Check sheet for the modelled part. Datum: model origin and axes. Units: mm. Round coordinates to 2 decimals unless told otherwise and drop trailing zeros. Loops run counter-clockwise (first coordinate to the right, second up) from the corner with the lowest first, then second, coordinate; pieces in that order, holes last. Notation, with made-up numbers: (41.5, 0) - (49.5, 0) arc R17 cw to (49.5, 29) - close; hole circle Ø11 at (-9.5, 38.25). An arc over 180 degrees is marked (long way). Put each result on its own line as item: value. Start each with the question number.
Item 1: Material ranges on line 1 along X through (y, z) = (2.9, 110); line 2 along X through (y, z) = (11.75, 110); line 3 along Z through (x, y) = (235, 3.95), recorded low to high.
Item 2: Section check B-B, the plane x = 169.5. Record the cut outline in (y, z), and give its area (3 significant figures).
Item 3: Section check C-C, the plane z = 136. Record the cut outline in (x, y).
Item 4: Section check A-A, the plane y = 12.75. Give the number of separate pieces and of enclosed holes in the cut face, and give its area (3 significant figures).
Item 5: Gauge pin test, flat ends, axial feed: pin 1 Ø8 at (x, z) = (-110, 155) entering from -Y; pin 2 Ø6.5 at (x, z) = (-205, 250) entering from +Y; pin 3 Ø10 at (x, z) = (-250, 155) entering from +Y; pin 4 Ø8 at (y, z) = (15.5, 198) entering from +X. Record the tip position at first contact, or that the pin passes through.
from build123d import *

# Parameters (mm, degrees)
SKETCH1_W                      = 520
SKETCH1_H                      = 200
BOSS_EXTRUDE1_DEPTH            = 20
SKETCH6_W                      = 160
SKETCH6_H                      = 160
BOSS_EXTRUDE2_DEPTH            = 20
CBORE_FOR_M6_SHCS1_AT_2_COUNT  = 2
CBORE_FOR_M6_SHCS1_AT_2_PITCH  = 150
CBORE_FOR_M6_SHCS1_AT_3_COUNT  = 2
CBORE_FOR_M6_SHCS1_AT_3_PITCH  = 470
CBORE_FOR_M6_SHCS1_AT_4_COUNT  = 2
CBORE_FOR_M6_SHCS1_AT_4_PITCH  = 493.355855342
CBORE_FOR_M6_SHCS1_AT_5_COUNT  = 2
CBORE_FOR_M6_SHCS1_AT_5_PITCH  = 75
CBORE_FOR_M6_SHCS1_AT_6_COUNT  = 2
CBORE_FOR_M6_SHCS1_AT_6_PITCH  = 475.946425556
CBORE_FOR_M6_SHCS1_AT_7_COUNT  = 2
CBORE_FOR_M6_SHCS1_AT_7_PITCH  = 507.666228934
CBORE_FOR_M6_SHCS1_AT_8_COUNT  = 2
CBORE_FOR_M6_SHCS1_AT_8_PITCH  = 547.014625033
CBORE_FOR_M6_SHCS1_AT_9_COUNT  = 2
CBORE_FOR_M6_SHCS1_AT_9_PITCH  = 431.653796462
CBORE_FOR_M6_SHCS1_AT_10_COUNT = 2
CBORE_FOR_M6_SHCS1_AT_10_PITCH = 477.310171691
CBORE_FOR_M6_SHCS1_AT_11_COUNT = 2
CBORE_FOR_M6_SHCS1_AT_11_PITCH = 414.638396678
CBORE_FOR_M6_SHCS1_AT_12_COUNT = 2
CBORE_FOR_M6_SHCS1_AT_12_PITCH = 536.77276384
CBORE_FOR_M6_SHCS1_AT_13_COUNT = 2
CBORE_FOR_M6_SHCS1_AT_13_PITCH = 560.022320984
CBORE_FOR_M6_SHCS1_AT_14_COUNT = 2
CBORE_FOR_M6_SHCS1_AT_14_PITCH = 444.325331261


with BuildPart() as part:
    # Sketch1 → Boss-Extrude1 (new body)
    with BuildSketch(Plane(origin=(0, 0, 0), x_dir=(1, 0, 0), z_dir=(0, 1, 0))):
        Rectangle(SKETCH1_W, SKETCH1_H)
    extrude(amount=BOSS_EXTRUDE1_DEPTH)

    # Sketch6 → Boss-Extrude2 (add)
    with BuildSketch(Plane.XZ):
        with Locations((-180, 180)):
            Rectangle(SKETCH6_W, SKETCH6_H)
    extrude(amount=-BOSS_EXTRUDE2_DEPTH)

    # Sketch5 → CBORE for M6 SHCS1 (revolve, cut)
    with BuildSketch(Plane(origin=(235, 0, -75), x_dir=(0, 0, -1), z_dir=(1, 0, 0))):
        Polygon((0, 0), (0, 20), (3.5, 20), (3.5, 6), (5.5, 6), (5.5, 0.020977491), (5.525, 0), align=None)
    cbore_for_m6_shcs1 = revolve(axis=Axis((235, -6.35, -75), (0, 1, 0)), mode=Mode.SUBTRACT)

    # CBORE for M6 SHCS1 at 2: CBORE for M6 SHCS1 ×2
    with Locations(*[(0, 0, i * CBORE_FOR_M6_SHCS1_AT_2_PITCH) for i in range(1, CBORE_FOR_M6_SHCS1_AT_2_COUNT)]):
        add(cbore_for_m6_shcs1, mode=Mode.SUBTRACT)

    # CBORE for M6 SHCS1 at 3: CBORE for M6 SHCS1 ×2
    with Locations(*[(-i * CBORE_FOR_M6_SHCS1_AT_3_PITCH, 0, 0) for i in range(1, CBORE_FOR_M6_SHCS1_AT_3_COUNT)]):
        add(cbore_for_m6_shcs1, mode=Mode.SUBTRACT)

    # CBORE for M6 SHCS1 at 4: CBORE for M6 SHCS1 ×2
    with Locations(*[Vector(-0.9526592112186828, 0, 0.30404017379319653) * (i * CBORE_FOR_M6_SHCS1_AT_4_PITCH) for i in range(1, CBORE_FOR_M6_SHCS1_AT_4_COUNT)]):
        add(cbore_for_m6_shcs1, mode=Mode.SUBTRACT)

    # CBORE for M6 SHCS1 at 5: CBORE for M6 SHCS1 ×2
    with Locations(*[(0, 0, i * CBORE_FOR_M6_SHCS1_AT_5_PITCH) for i in range(1, CBORE_FOR_M6_SHCS1_AT_5_COUNT)]):
        add(cbore_for_m6_shcs1, mode=Mode.SUBTRACT)

    # CBORE for M6 SHCS1 at 6: CBORE for M6 SHCS1 ×2
    with Locations(*[Vector(-0.9875061031301207, 0, 0.15758076113778519) * (i * CBORE_FOR_M6_SHCS1_AT_6_PITCH) for i in range(1, CBORE_FOR_M6_SHCS1_AT_6_COUNT)]):
        add(cbore_for_m6_shcs1, mode=Mode.SUBTRACT)

    # CBORE for M6 SHCS1 at 7: CBORE for M6 SHCS1 ×2
    with Locations(*[Vector(-0.7682212795973759, 0, 0.6401843996644799) * (i * CBORE_FOR_M6_SHCS1_AT_7_PITCH) for i in range(1, CBORE_FOR_M6_SHCS1_AT_7_COUNT)]):
        add(cbore_for_m6_shcs1, mode=Mode.SUBTRACT)

    # CBORE for M6 SHCS1 at 8: CBORE for M6 SHCS1 ×2
    with Locations(*[Vector(-0.8043660623762138, 0, 0.594134023346067) * (i * CBORE_FOR_M6_SHCS1_AT_8_PITCH) for i in range(1, CBORE_FOR_M6_SHCS1_AT_8_COUNT)]):
        add(cbore_for_m6_shcs1, mode=Mode.SUBTRACT)

    # CBORE for M6 SHCS1 at 9: CBORE for M6 SHCS1 ×2
    with Locations(*[Vector(-0.9035018415143107, 0, 0.42858420687217297) * (i * CBORE_FOR_M6_SHCS1_AT_9_PITCH) for i in range(1, CBORE_FOR_M6_SHCS1_AT_9_COUNT)]):
        add(cbore_for_m6_shcs1, mode=Mode.SUBTRACT)

    # CBORE for M6 SHCS1 at 10: CBORE for M6 SHCS1 ×2
    with Locations(*[Vector(-0.9218324395662549, 0, 0.3875886393630844) * (i * CBORE_FOR_M6_SHCS1_AT_10_PITCH) for i in range(1, CBORE_FOR_M6_SHCS1_AT_10_COUNT)]):
        add(cbore_for_m6_shcs1, mode=Mode.SUBTRACT)

    # CBORE for M6 SHCS1 at 11: CBORE for M6 SHCS1 ×2
    with Locations(*[Vector(-0.8320502943378436, 0, 0.5547001962252293) * (i * CBORE_FOR_M6_SHCS1_AT_11_PITCH) for i in range(1, CBORE_FOR_M6_SHCS1_AT_11_COUNT)]):
        add(cbore_for_m6_shcs1, mode=Mode.SUBTRACT)

    # CBORE for M6 SHCS1 at 12: CBORE for M6 SHCS1 ×2
    with Locations(*[Vector(-0.9035480796952873, 0, 0.42848671820601264) * (i * CBORE_FOR_M6_SHCS1_AT_12_PITCH) for i in range(1, CBORE_FOR_M6_SHCS1_AT_12_COUNT)]):
        add(cbore_for_m6_shcs1, mode=Mode.SUBTRACT)

    # CBORE for M6 SHCS1 at 13: CBORE for M6 SHCS1 ×2
    with Locations(*[Vector(-0.8660369092932877, 0, 0.49998007134457856) * (i * CBORE_FOR_M6_SHCS1_AT_13_PITCH) for i in range(1, CBORE_FOR_M6_SHCS1_AT_13_COUNT)]):
        add(cbore_for_m6_shcs1, mode=Mode.SUBTRACT)

    # CBORE for M6 SHCS1 at 14: CBORE for M6 SHCS1 ×2
    with Locations(*[Vector(-0.7764580943901146, 0, 0.6301688882006727) * (i * CBORE_FOR_M6_SHCS1_AT_14_PITCH) for i in range(1, CBORE_FOR_M6_SHCS1_AT_14_COUNT)]):
        add(cbore_for_m6_shcs1, mode=Mode.SUBTRACT)


solid = part.part
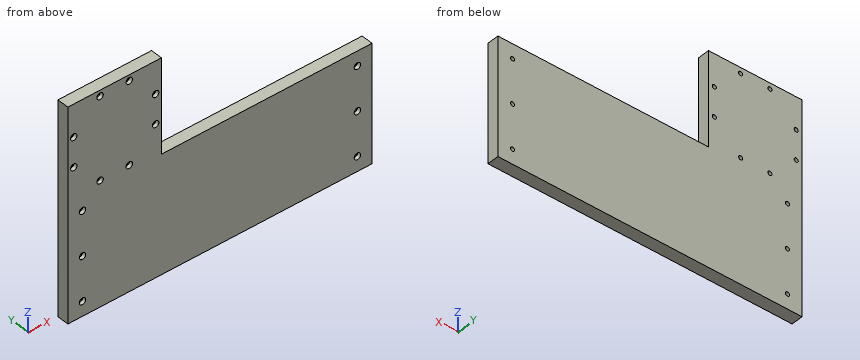
Check result:
1. line 1: -260 to -210.5, -199.5 to -160.5, -149.5 to -100
1. line 2: -260 to -208.5, -201.5 to -158.5, -151.5 to -100
1. line 3: -100 to -80.5, -69.5 to -5.5, 5.5 to 69.5, 80.5 to 100
2. outline: (0, -100) - (20, -100) - (20, 100) - (0, 100) - close
2. area: 4,000 mm²
3. outline: (-260, 0) - (-100, 0) - (-100, 20) - (-260, 20) - close
4. separate pieces: 1
4. enclosed holes: 14
4. area: 129,000 mm²
5. pin 1: y = 6
5. pin 2: through
5. pin 3: y = 20
5. pin 4: x = -100
